Source: CAD feature listing. Evaluate the final solid. Frame: model axes, mm. Round coordinates to 2 decimals unless told otherwise and drop trailing zeros. Order: outer loops, then holes, each group sorted by start corner. A loop starts at its lowest first (then second) coordinate and runs counter-clockwise, first axis right, second up.
```python
from build123d import *

# Parameters (mm, degrees)
SKETCH1_W           = 87.5284
SKETCH1_H           = 45.72
SKETCH1_W_2         = 19.05
SKETCH1_H_2         = 2.7432
BOSS_EXTRUDE1_DEPTH = 2.7432
SKETCH2_W           = 2.7432
SKETCH2_H           = 19.05
SKETCH2_W_2         = 19.05
SKETCH2_H_2         = 2.7432
CUT_EXTRUDE1_DEPTH  = 3.7432


with BuildPart() as part:
    # Sketch1 → Boss-Extrude1 (new body)
    with BuildSketch(Plane.XY):
        Rectangle(SKETCH1_W, SKETCH1_H)
        with Locations((0, -14.7066)):
            Rectangle(SKETCH1_W_2, SKETCH1_H_2, mode=Mode.SUBTRACT)
    extrude(amount=BOSS_EXTRUDE1_DEPTH)

    # Sketch2 → Cut-Extrude1 (cut, through all)
    with BuildSketch(Plane.XY.offset(2.7432)):
        with Locations((-42.3926, 0)):
            Rectangle(SKETCH2_W, SKETCH2_H)
        with Locations((42.3926, 0)):
            Rectangle(SKETCH2_W, SKETCH2_H)
        with Locations((0, 21.4884)):
            Rectangle(SKETCH2_W_2, SKETCH2_H_2)
    extrude(amount=-CUT_EXTRUDE1_DEPTH, mode=Mode.SUBTRACT)


solid = part.part
```
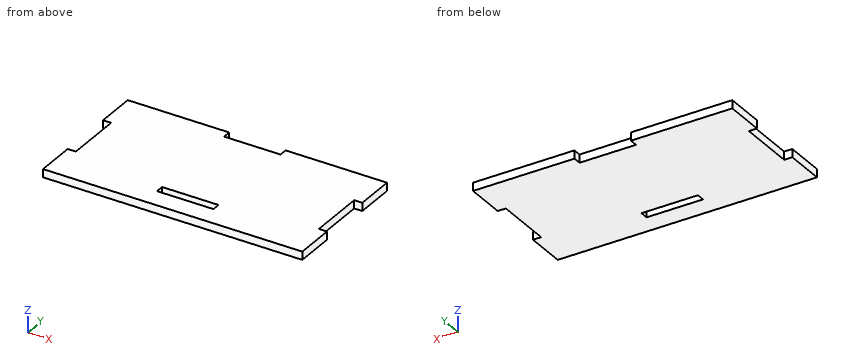
1. Section A-A on z = 2.1. Return loops of the section in (x, y) (3 decimals), plus the area to 3 significant figures.
2. Line query: line 1 along Y through (x, z) = (8, 1.95) (3 decimals); line 2 along X through (y, z) = (-5, 0.45). Output: solid intervals per line, ascending.
3. Section B-B on y = 6.5. Return loops of the section in (x, z), plus the area to 3 significant figures.
4. First-contact query: pin 1 (0.8 mm diameter, centred on y = -3.5, z = 1.5, fed in from +X). Flat tip, straight axial feed; report the tip coordinate or a pass-through.
Result:
1. outline: (-43.764, -22.86) - (43.764, -22.86) - (43.764, -9.525) - (41.021, -9.525) - (41.021, 9.525) - (43.764, 9.525) - (43.764, 22.86) - (9.525, 22.86) - (9.525, 20.117) - (-9.525, 20.117) - (-9.525, 22.86) - (-43.764, 22.86) - (-43.764, 9.525) - (-41.021, 9.525) - (-41.021, -9.525) - (-43.764, -9.525) - close; hole (-9.525, -16.078) - (9.525, -16.078) - (9.525, -13.335) - (-9.525, -13.335) - close
1. area: 3,790 mm2
2. line 1: y = -22.86 to -16.078, -13.335 to 20.117
2. line 2: x = -41.02 to 41.02
3. outline: (-41.02, 0) - (41.02, 0) - (41.02, 2.74) - (-41.02, 2.74) - close
3. area: 225 mm2
4. pin 1: stops at x = 41.02
